Autodesk Inventor part; units mm, degrees
ref_plane "Start Plane" through (0, 0, 25) normal (0, 0, 1) x (1, 0, 0)
ref_plane "End Plane" through (0, 0, 334.9974) normal (0, 0, 1) x (1, 0, 0)
ref_plane "Work Plane4" through (1275, 21, 25) normal (0, 0, -1) x (-1, 0, 0)
ref_plane "Start Plane" through (0, 0, 25) normal (0, 0, 1) x (1, 0, 0)
ref_plane "End Plane" through (0, 0, 334.9974) normal (0, 0, 1) x (1, 0, 0)
sketch "Sketch" plane through (0, 0, 0) normal (0, 0, 1) x (1, 0, 0)
  line L0 (-25, -21) -> (-25, 21)
  line L1 (-21, 25) -> (21, 25)
  line L2 (25, 21) -> (25, -21)
  line L3 (21, -25) -> (-21, -25)
  arc A0 (-25, -21) -> (-21, -25) centre (-21, -21) ccw
  arc A1 (25, 21) -> (21, 25) centre (21, 21) ccw
  arc A2 (-21, 25) -> (-25, 21) centre (-21, 21) ccw
  arc A3 (21, -25) -> (25, -21) centre (21, -21) ccw
  arc A4 (-21, 23) -> (-23, 21) centre (-21, 21) ccw
  line L4 (-21, 23) -> (21, 23)
  arc A5 (23, 21) -> (21, 23) centre (21, 21) ccw
  line L5 (23, 21) -> (23, -21)
  arc A6 (21, -23) -> (23, -21) centre (21, -21) ccw
  line L6 (21, -23) -> (-21, -23)
  arc A7 (-23, -21) -> (-21, -23) centre (-21, -21) ccw
  line L7 (-23, -21) -> (-23, 21)
  line L8 (0, 36.1598) -> (0, -36.1598) construction
  line L9 (-36.1598, 0) -> (36.1598, 0) construction
  dimension "d7" = 4
  dimension "d9" = 50
  dimension "d11" = 50
  dimension "d12" = 2
  dimension "d15" = 25
  dimension "d16" = 25
extrude "Body" add sketch "Sketch" along normal up to surface (309.9974 mm away) from surface at 25
sketch "Sketch3" plane through (0, 0, 0) normal (0, 0, 1) x (1, 0, 0)
  line L0 (0, 0) -> (10, 0)
ref_plane "Work Plane3" through (0, 0, 0) normal (0, -1, 0) x (1, 0, 0)
sketch "Sketch4" plane through (0, 0, 0) normal (0, -1, 0) x (1, 0, 0)
  line L0 (-2, 25) -> (12, 25)
  line L1 (-2, 334.9974) -> (12, 334.9974)
  dimension "d18" = 309.9974
ref_plane "Work Plane4" through (1275, 21, 25) normal (0, 0, -1) x (-1, 0, 0)
split "Split1" plane through (1275, 21, 25) removes the side toward (0, 0, -1)
ref_plane "Work Plane5" through (-1042.5, 21, 334.9974) normal (0, 0, 1) x (1, 0, 0)
split "Split2" plane through (-1042.5, 21, 334.9974) removes the side toward (0, 0, 1)
ref_plane "Work Plane6" through (1270, -21, 785) normal (0, 0, 1) x (1, 0, 0)
split "Split3" plane through (1270, -21, 785) removes the side toward (0, 0, 1)
equation "\"d7\" = G_IR"
equation "\"d9\" = G_W"
equation "\"d11\" = G_H"
equation "\"d12\" = G_T"
equation "\"d15\" = 0.5 * d9"
equation "\"d16\" = 0.5 * d11"
equation "\"d3\" = G_L"
equation "\"G_W\" = 50"
equation "\"G_H\" = 50"
equation "\"G_T\" = 2"
equation "\"G_IR\" = 4"
equation "\"G_L\" = d18"
equation "\"G_OFFSET_START\" = -25"
equation "\"G_OFFSET_END\" = 124.9974"
equation "\"d13\" = -G_OFFSET_START"
equation "\"d14\" = G_OFFSET_END + B_L"
properties part number "ISO 10799-2 - 50x50x2 - 310" material "Steel, Galvanized"
Work out the finished part from the listing and answer in its coordinate system (mm). A direction names the side the tool comes from. Round coordinates to 2 decimals unless told otherwise and drop trailing zeros. Write each loop counter-clockwise with the first axis right and the second up, starting at its lowest first coordinate (ties: lowest second). Pieces come first, ordered by that corner, then holes.
1) The mould has two halves that part along X. Classify faces 1 (the flat face through (0, 24, 25)), 2 (the flat face through (0, 23, 178)), 3 (the flat face through (-25, 0, 178)): pulls with the +X half, pulls with the -X half, needs draft (parallel to the pull), parting line crosses it, or undercut.
2) A cutting plane is placed at C-C (z = 169). Give the vertices of the cut face in (x, y).
3) A tool of negligible diameter and unlimited length cuts with its end or side. For faces 4 (the flat face through (-23, 0, 178)), 5 (the flat face through (0, -25, 178)), from which of +Z, -Z, +X, -X, +Y, -Y can it reach the whole face along a straight path? Write none if from no direction.
4) A cutting plane is placed at A-A (x = -10.5). Give the vertices of the cut face in (y, z).
5) Straight lines are drawn through the part: line 1 (Y direction, x = -3, z = 124); line 2 (Y direction, x = 22, z = 89). For each, find the intervals that lie inside material, in ascending order.
Completed:
1. face 1: needs draft
1. face 2: undercut
1. face 3: pulls with the -X half
2. outline: (-25, -21) arc R4 ccw to (-21, -25) - (21, -25) arc R4 ccw to (25, -21) - (25, 21) arc R4 ccw to (21, 25) - (-21, 25) arc R4 ccw to (-25, 21) - close; hole (-23, -21) arc R2 ccw to (-21, -23) - (21, -23) arc R2 ccw to (23, -21) - (23, 21) arc R2 ccw to (21, 23) - (-21, 23) arc R2 ccw to (-23, 21) - close
3. face 4: +Z, -Z
3. face 5: +Z, -Z, +X, -X, -Y
4. outline: (-25, 25) - (-23, 25) - (-23, 335) - (-25, 335) - close; (23, 25) - (25, 25) - (25, 335) - (23, 335) - close
5. line 1: y = -25 to -23, 23 to 25
5. line 2: y = -24.87 to -22.73, 22.73 to 24.87
